```python
from build123d import *

# Parameters (mm, degrees)
ESBO_O1_W                                    = 75
ESBO_O1_H                                    = 35
RESSALTO_EXTRUS_O1_DEPTH                     = 20
ESBO_O2_R                                    = 10.5
ESBO_O2_R_2                                  = 5.15
CORTE_EXTRUS_O1_DEPTH                        = 21
ESBO_O3_R                                    = 11
CORTE_EXTRUS_O2_DEPTH                        = 4
FURO_ROSCADO_PARA_CONDU_TE_DE_M3X0_51_D      = 3.15
FURO_ROSCADO_PARA_CONDU_TE_DE_M3X0_51_DEPTH  = 10
FURO_ROSCADO_PARA_CONDU_TE_DE_M3X0_51_TIP    = 0.946355475
FURO_ROSCADO_PARA_CONDU_TE_DE_5_16_241_D     = 8.33374
FURO_ROSCADO_PARA_CONDU_TE_DE_5_16_241_DEPTH = 12
FURO_ROSCADO_PARA_CONDU_TE_DE_5_16_241_TIP   = 2.503708088


with BuildPart() as part:
    # Esboço1 → Ressalto-extrusão1 (new body)
    with BuildSketch(Plane.XY):
        Rectangle(ESBO_O1_W, ESBO_O1_H)
    extrude(amount=RESSALTO_EXTRUS_O1_DEPTH)

    # Esboço2 → Corte-extrusão1 (cut, through all)
    with BuildSketch(Plane.XY.offset(20)):
        with Locations((-24, -5)):
            Circle(ESBO_O2_R)
        with Locations((0, -5)):
            Circle(ESBO_O2_R_2)
        with Locations((24, -5)):
            Circle(ESBO_O2_R)
    extrude(amount=-CORTE_EXTRUS_O1_DEPTH, mode=Mode.SUBTRACT)

    # Esboço3 → Corte-extrusão2 (cut)
    with BuildSketch(Plane.XY.offset(20)):
        with Locations((0, -5)):
            Circle(ESBO_O3_R)
    extrude(amount=-CORTE_EXTRUS_O2_DEPTH, mode=Mode.SUBTRACT)

    # Furo roscado para conduíte de M3x0.51
    with Locations(Plane.XY.offset(16)):
        with Locations((-8, -5.125635555), (-0.125635555, 3), (8, -4.874364445), (0.125635555, -13)):
            Hole(FURO_ROSCADO_PARA_CONDU_TE_DE_M3X0_51_D / 2, depth=FURO_ROSCADO_PARA_CONDU_TE_DE_M3X0_51_DEPTH)
            with Locations((0, 0, -(FURO_ROSCADO_PARA_CONDU_TE_DE_M3X0_51_DEPTH + FURO_ROSCADO_PARA_CONDU_TE_DE_M3X0_51_TIP / 2))):  # 118° drill point
                Cone(0, FURO_ROSCADO_PARA_CONDU_TE_DE_M3X0_51_D / 2, FURO_ROSCADO_PARA_CONDU_TE_DE_M3X0_51_TIP, mode=Mode.SUBTRACT)

    # Furo roscado para conduíte de 5/16-241
    with Locations(Plane(origin=(0, 17.5, 0), x_dir=(1, 0, 0), z_dir=(0, 1, 0))):
        with Locations((-12, -10), (12, -10)):
            Hole(FURO_ROSCADO_PARA_CONDU_TE_DE_5_16_241_D / 2, depth=FURO_ROSCADO_PARA_CONDU_TE_DE_5_16_241_DEPTH)
            with Locations((0, 0, -(FURO_ROSCADO_PARA_CONDU_TE_DE_5_16_241_DEPTH + FURO_ROSCADO_PARA_CONDU_TE_DE_5_16_241_TIP / 2))):  # 118° drill point
                Cone(0, FURO_ROSCADO_PARA_CONDU_TE_DE_5_16_241_D / 2, FURO_ROSCADO_PARA_CONDU_TE_DE_5_16_241_TIP, mode=Mode.SUBTRACT)


solid = part.part
```
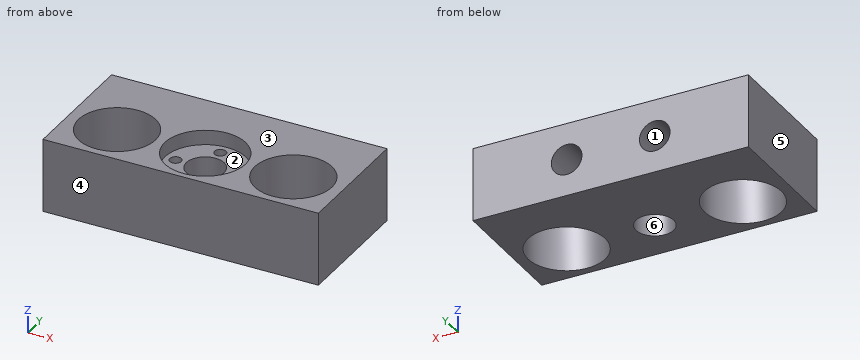
Check sheet for the modelled part. Datum: model origin and axes. Units: mm. Face numbers are marked on the shaded views. A direction names the side the tool comes from. Round coordinates to 2 decimals unless told otherwise and drop trailing zeros. Order: outer loops, then holes, each group sorted by start corner. A loop starts at its lowest first (then second) coordinate and runs counter-clockwise, first axis right, second up. Notation, with made-up numbers: (49, 48.5) -> (53, 48.5) arc R30 ccw to (53, 81.5) -> close; hole circle Ø11 at (82, 69). An arc over 180 degrees is marked (long way). One line per item, written item: value. Start each with the question number.
Q1. Cross-section at B-B (y = 11). Record the boundary of the cut face in (x, z), and give its area (3 significant figures).
Q2. Cross-section at D-D (z = 13). Give the number of separate pieces and of enclosed holes in the cut face, and give its area (3 significant figures).
Q3. Set-up check for the marked faces 1, 2 and 3: record each of +Z, -Z, +X, -X, +Y, -Y from which the full face is reachable in a straight line by a thin tool's end or side.
Q4. Cross-section at A-A (x = 24). Record the boundary of the cut face in (y, z).
Q5. Mould release check, pull along Y, two halves, no side actions. Record for the marked faces 4, 5 and 6: pulls with the +Y half, pulls with the -Y half, needs draft (parallel to the pull), parting line crosses it, or undercut.
Q6. Gauge pin test, flat ends, axial feed: pin 1 Ø6.5 at (x, z) = (12, 10) entering from +Y; pin 2 Ø3.5 at (x, y) = (-8, -5.13) entering from +Z. Record the tip position at first contact, or that the pin passes through.
Q7. Cross-section at C-C (x = -3). Record the boundary of the cut face in (y, z), and give its area (3 significant figures).
Q8. Thickness scan on line 1 (Y direction, x = 0, z = 11); line 2 (Y direction, x = 0, z = 17.45); line 3 (X direction, y = 12.5, z = 9.25). Record the ranges inside material, lowest first.
Completed:
1. outline: (-37.5, 0) -> (37.5, 0) -> (37.5, 20) -> (-37.5, 20) -> close; hole circle Ø8.33 at (-12, 10); hole circle Ø8.33 at (12, 10)
1. area: 1,390 mm²
2. separate pieces: 1
2. enclosed holes: 7
2. area: 1,670 mm²
3. face 1: +Y
3. face 2: +Z
3. face 3: +Z, +X, -X, +Y, -Y
4. outline: (-17.5, 0) -> (-15.5, 0) -> (-15.5, 20) -> (-17.5, 20) -> close; (5.5, 0) -> (17.5, 0) -> (17.5, 20) -> (5.5, 20) -> close
5. face 4: pulls with the -Y half
5. face 5: needs draft
5. face 6: undercut
6. pin 1: stops at y = 4.95
6. pin 2: stops at z = 16
7. outline: (-17.5, 0) -> (-9.19, 0) -> (-9.19, 16) -> (-15.58, 16) -> (-15.58, 20) -> (-17.5, 20) -> close; (-0.81, 0) -> (17.5, 0) -> (17.5, 20) -> (5.58, 20) -> (5.58, 16) -> (-0.81, 16) -> close
7. area: 481 mm²
8. line 1: y = -17.5 to -14.57, -11.43 to -10.15, 0.15 to 1.43, 4.57 to 17.5
8. line 2: y = -17.5 to -16, 6 to 17.5
8. line 3: x = -37.5 to -16.1, -7.9 to 7.9, 16.1 to 37.5
